Autodesk Inventor part; units mm, degrees
ref_plane "Work Plane1" through (0, 0, -4) normal (0, 0, 1) x (1, 0, 0)
ref_plane "YZ Plane" through (0, 0, 0) normal (1, 0, 0) x (0, 1, 0)
ref_plane "XZ Plane" through (0, 0, 0) normal (0, 1, 0) x (-1, 0, 0)
sketch "Sketch1" plane through (0, 0, 0) normal (1, 0, 0) x (0, 1, 0)
  arc A0 (-0.9778, 3.8786) -> (1.0222, 3.8672) centre (0, 0) ccw
  circle A1 centre (0, 0) radius 4
  dimension "d0" = 8
extrude "Extrusion1" add sketch "Sketch1" against normal blind 105
sketch "Sketch2" plane through (0, 0, 0) normal (0, 0, 1) x (1, 0, 0)
  line L0 (-2.44, 6.5) -> (-1.5, 6.5)
  line L1 (-1.5, 6.5) -> (-1.5, 3.5)
  line L2 (-1.5, 3.5) -> (-2.44, 3.5)
  line L3 (-2.44, 3.5) -> (-2.44, 6.5)
  line L4 (0, 4) -> (0, -4)
  line L5 (0, 4) -> (-105, 4)
  line L6 (-126, 0) -> (21, 0)
  line L7 (0, 4) -> (-105, 4)
  line L8 (-52.5, 4) -> (-52.5, -9.5088)
  line L9 (-102.56, 6.5) -> (-103.5, 6.5)
  line L10 (-103.5, 6.5) -> (-103.5, 3.5)
  line L11 (-103.5, 3.5) -> (-102.56, 3.5)
  line L12 (-102.56, 3.5) -> (-102.56, 6.5)
  line L13 (-105, 4) -> (-105, -4)
  line L14 (0, -4) -> (-105, -4)
  point P0 (0, 0)
  point P1 (0, 1.0222)
  point P2 (0, -0.9778)
  point P3 (-105, 0)
  point P4 (-105, 1.0222)
  point P5 (-105, -0.9778)
  dimension "d9" = 1.5
  dimension "d10" = 0.94
  dimension "d11" = 0.5
  dimension "d12" = 3
  dimension "d18" = 8
revolve "Revolution1" cut sketch "Sketch2" angle 360 about axis through (-10, 0, 0) along (1, 0, 0) contours L0 L1 L5 L3 | L5 L1 L2 L3 | L12 L11 L10 L5 | L5 L10 L9 L12
ref_plane "Work Plane1" through (0, 0, -4) normal (0, 0, 1) x (1, 0, 0)
sketch "Sketch5" plane through (0, 0, -4) normal (0, 0, 1) x (1, 0, 0)
  line L0 (-73, 1) -> (-55, 1)
  line L1 (-55, 1) -> (-55, -1)
  line L2 (-55, -1) -> (-73, -1)
  line L3 (-73, -1) -> (-73, 1)
  line L4 (-2.44, -4) -> (-102.56, -4)
  line L5 (-2.44, 4) -> (-102.56, 4)
  line L6 (-105, 4) -> (-105, -4)
  circle A0 centre (-55, 0) radius 1
  circle A1 centre (-73, 0) radius 1
  line L7 (-42.5, 1) -> (-24.5, 1)
  line L8 (-24.5, 1) -> (-24.5, -1)
  line L9 (-24.5, -1) -> (-42.5, -1)
  line L10 (-42.5, -1) -> (-42.5, 1)
  circle A2 centre (-24.5, 0) radius 1
  circle A3 centre (-42.5, 0) radius 1
  line L11 (0, 4) -> (0, -4)
  point P0 (0, 0)
  dimension "d24" = 20
  dimension "d19" = 2
  dimension "d20" = 8
  dimension "d21" = 3
  dimension "d22" = 32
  dimension "d23" = 18
  dimension "d25" = 2
  dimension "d26" = 24.5
  dimension "d27" = 18
extrude "Extrusion4" cut sketch "Sketch5" along normal blind 1.2
equation "\"d21\" = 0.5 * d20 - 0.5 * d19"
properties part number "AxeHorizontalRoller" material "Stainless Steel"
The listing builds one solid part. Answer for the finished solid, in the listing's coordinates (mm). A direction names the side the tool comes from. Round coordinates to 2 decimals unless told otherwise and drop trailing zeros. Write each loop counter-clockwise with the first axis right and the second up, starting at its lowest first coordinate (ties: lowest second). Pieces come first, ordered by that corner, then holes. Notation, with made-up numbers: (66, 9.25) -> (109, 9.25) arc R17 ccw to (109, 22.25) -> close; hole circle Ø3 at (49, -39.75). An arc over 180 degrees is marked (long way). Answer as a JSON object with one key per item and string values. Group by question number.
Q1. Section D-D (x = -97.5) is taken. Write down the section's boundary in (y, z).
Q2. Which of the six approach directions +Z, -Z, +X, -X, +Y, -Y give full straight-line access (tool end or side, diameter ignored) to faces 1 (the face through (-64, 0, -2.8)), 2 (the face through (-104, 0, -4)), 3 (the face through (-103.023, 3.233, -1.341))?
Q3. Section A-A (y = 0) is taken. Write down the section's boundary in (x, z), plus the area to 3 significant figures.
Q4. Section B-B (z = 2.5) is taken. Write down the section's boundary in (x, y).
Q5. Determine the mould class of faces 4 (the face through (-52, 0, -4)), 5 (the face through (-105, 0, 0)), 6 (the face through (-34, 0, -2.8)) for opening direction X: pulls with the +X half, pulls with the -X half, needs draft (parallel to the pull), parting line crosses it, or undercut.
Q6. Straight lines are drawn through the part: line 1 along X through (y, z) = (3.75, -1); line 2 along X through (y, z) = (0.25, -3.25); line 3 along Z through (x, y) = (-75.5, -0.25). For each, find the intervals that lie inside material, in ascending order.
Q7. Section C-C (x = -29) is taken. Write down the section's boundary in (y, z).
Q8. Each of these flat-tipped pins is pushed along its axis until it touches: pin 1 Ø2 at (x, z) = (-61, 2.5) entering from +Y; pin 2 Ø4 at (x, y) = (-61.5, 2) entering from -Z; pin 3 Ø1 at (x, y) = (-32.5, 0) entering from -Z. Where does it stop, or does it pass through?
Check values:
{
 "1": {"outline": "(-0.98, 3.88) arc R4 ccw (long way) to (1.02, 3.87) arc R4 ccw to start"},
 "2": {"face 1": "-Z", "face 2": "+X, -X", "face 3": "none"},
 "3": {"outline": "(-105, -4) -> (-103.5, -4) -> (-103.5, -3.5) -> (-102.56, -3.5) -> (-102.56, -4) -> (-74, -4) -> (-74, -2.8) -> (-54, -2.8) -> (-54, -4) -> (-43.5, -4) -> (-43.5, -2.8) -> (-23.5, -2.8) -> (-23.5, -4) -> (-2.44, -4) -> (-2.44, -3.5) -> (-1.5, -3.5) -> (-1.5, -4) -> (0, -4) -> (0, 4) -> (-1.5, 4) -> (-1.5, 3.5) -> (-2.44, 3.5) -> (-2.44, 4) -> (-102.56, 4) -> (-102.56, 3.5) -> (-103.5, 3.5) -> (-103.5, 4) -> (-105, 4) -> close", "area": "790 mm^2"},
 "4": {"outline": "(-105, -3.12) -> (-103.5, -3.12) -> (-103.5, -2.45) -> (-102.56, -2.45) -> (-102.56, -3.12) -> (-2.44, -3.12) -> (-2.44, -2.45) -> (-1.5, -2.45) -> (-1.5, -3.12) -> (0, -3.12) -> (0, 3.12) -> (-1.5, 3.12) -> (-1.5, 2.45) -> (-2.44, 2.45) -> (-2.44, 3.12) -> (-102.56, 3.12) -> (-102.56, 2.45) -> (-103.5, 2.45) -> (-103.5, 3.12) -> (-105, 3.12) -> close"},
 "5": {"face 4": "needs draft", "face 5": "pulls with the -X half", "face 6": "undercut"},
 "6": {"line 1": "-105 to -103.5, -102.56 to -2.44, -1.5 to 0", "line 2": "-105 to -73.97, -54.03 to -43.47, -23.53 to 0", "line 3": "-3.99 to 3.99"},
 "7": {"outline": "(-1, -3.87) -> (-1, -2.8) -> (1, -2.8) -> (1, -3.87) arc R4 ccw to (1.02, 3.87) arc R4 ccw to (-0.98, 3.88) arc R4 ccw to start"},
 "8": {"pin 1": "y = 3.71", "pin 2": "z = -3.87", "pin 3": "z = -2.8"}
}
